```python
from build123d import *

# Parameters (mm, degrees)
SKETCH1_W           = 106
SKETCH1_H           = 106
BOSS_EXTRUDE1_DEPTH = 10
CUT_EXTRUDE9_DEPTH  = 1.5
SKETCH18_W          = 106
SKETCH18_H          = 106
SKETCH18_W_2        = 100
SKETCH18_H_2        = 100
CUT_EXTRUDE14_DEPTH = 10
SKETCH20_R          = 1
CUT_EXTRUDE15_DEPTH = 8
CUT_EXTRUDE16_START = -8
SKETCH21_R          = 1
CUT_EXTRUDE16_DEPTH = 8
SKETCH23_W          = 100
SKETCH23_H          = 100
SKETCH23_W_2        = 98
SKETCH23_H_2        = 98
CUT_EXTRUDE17_DEPTH = 10
SKETCH17_W          = 26.25282414
SKETCH17_H          = 10
CUT_EXTRUDE19_DEPTH = 10
FILLET2_R           = 3
FILLET3_R           = 3
FILLET4_R           = 2
SKETCH26_R          = 1.5
CUT_EXTRUDE20_DEPTH = 10
SKETCH27_R          = 2.5
CUT_EXTRUDE21_DEPTH = 2


with BuildPart() as part:
    # Sketch1 → Boss-Extrude1 (new body)
    with BuildSketch(Plane(origin=(0, 0, 0), x_dir=(1, 0, 0), z_dir=(0, 1, 0))):
        Rectangle(SKETCH1_W, SKETCH1_H)
    extrude(amount=BOSS_EXTRUDE1_DEPTH)

    # Sketch12 → Cut-Extrude9 (cut)
    with BuildSketch(Plane(origin=(53, 0, 0), x_dir=(0, 0, -1), z_dir=(1, 0, 0))):
        with BuildLine():
            ThreePointArc((-17.75, 5), (-18.262563133, 6.237436867), (-19.5, 6.75))
            Line((-19.5, 6.75), (-19.5, 3.25))
            ThreePointArc((-19.5, 3.25), (-18.262563133, 3.762563133), (-17.75, 5))
        make_face()
        with BuildLine():
            Line((-19.5, 3.25), (-19.5, 6.75))
            ThreePointArc((-19.5, 6.75), (-21.25, 5), (-19.5, 3.25))
        make_face()
        with BuildLine():
            ThreePointArc((21.25, 5), (20.737436867, 6.237436867), (19.5, 6.75))
            Line((19.5, 6.75), (19.5, 3.25))
            ThreePointArc((19.5, 3.25), (20.737436867, 3.762563133), (21.25, 5))
        make_face()
        with BuildLine():
            Line((19.5, 3.25), (19.5, 6.75))
            ThreePointArc((19.5, 6.75), (17.75, 5), (19.5, 3.25))
        make_face()
    extrude(amount=-CUT_EXTRUDE9_DEPTH, mode=Mode.SUBTRACT)

    # Sketch18 → Cut-Extrude14 (cut)
    with BuildSketch(Plane.XZ):
        Rectangle(SKETCH18_W, SKETCH18_H)
        Rectangle(SKETCH18_W_2, SKETCH18_H_2, mode=Mode.SUBTRACT)
    extrude(amount=-CUT_EXTRUDE14_DEPTH, mode=Mode.SUBTRACT)

    # Sketch20 → Cut-Extrude15 (cut)
    with BuildSketch(Plane(origin=(50, 0, 0), x_dir=(0, 0, -1), z_dir=(1, 0, 0))):
        with Locations((19.5, 5)):
            Circle(SKETCH20_R)
        with Locations((-19.5, 5)):
            Circle(SKETCH20_R)
    extrude(amount=-CUT_EXTRUDE15_DEPTH, mode=Mode.SUBTRACT)

    # Sketch21 → Cut-Extrude16 (cut)
    with BuildSketch(Plane.ZY.offset(50).offset(CUT_EXTRUDE16_START)):
        with Locations(Location((19.5, 5, 0), (0, 0, 180))):
            Circle(SKETCH21_R)
        with Locations(Location((-19.5, 5, 0), (0, 0, 180))):
            Circle(SKETCH21_R)
    extrude(amount=CUT_EXTRUDE16_DEPTH, mode=Mode.SUBTRACT)

    # Sketch23 → Cut-Extrude17 (cut)
    with BuildSketch(Plane.XZ):
        Rectangle(SKETCH23_W, SKETCH23_H)
        Rectangle(SKETCH23_W_2, SKETCH23_H_2, mode=Mode.SUBTRACT)
    extrude(amount=-CUT_EXTRUDE17_DEPTH, mode=Mode.SUBTRACT)

    # Sketch17 → Cut-Extrude19 (cut)
    with BuildSketch(Plane.XZ):
        Polygon((-40.464466094, 44), (0, 3.535533906), (40.464466094, 44), (17.869219367, 44), (17.869219367, 29), (-17.869219367, 29), (-17.869219367, 44), align=None)
        with Locations((0, 39)):
            Rectangle(SKETCH17_W, SKETCH17_H)
        Polygon((44, -40.464466094), (44, 40.464466094), (3.535533906, 0), align=None)
        Polygon((-3.535533906, 0), (-44, 40.464466094), (-44, -40.464466094), align=None)
        Polygon((17.869219367, -44), (40.464466094, -44), (0, -3.535533906), (-40.464466094, -44), (-17.869219367, -44), (-17.869219367, -29), (17.869219367, -29), align=None)
        with Locations((0, -39)):
            Rectangle(SKETCH17_W, SKETCH17_H)
    extrude(amount=-CUT_EXTRUDE19_DEPTH, mode=Mode.SUBTRACT)

    # Fillet2
    fillet2_edges = [part.edges().sort_by_distance(p)[0] for p in [
        (40.464466094, 5, 44),
        (0, 5, 3.535533906),
        (-40.464466094, 5, 44),
        (44, 5, 40.464466094),
        (3.535533906, 5, 0),
        (44, 5, -40.464466094),
        (-44, 5, -40.464466094),
        (-44, 5, 40.464466094),
        (-3.535533906, 5, 0),
        (-40.464466094, 5, -44),
        (0, 5, -3.535533906),
        (40.464466094, 5, -44),
    ]]
    fillet(fillet2_edges, radius=FILLET2_R)

    # Fillet3
    fillet3_edges = [part.edges().sort_by_distance(p)[0] for p in [
        (17.869219367, 5, 29),
        (17.869219367, 5, 44),
        (-17.869219367, 5, 44),
        (-17.869219367, 5, 29),
        (17.869219367, 5, -44),
        (17.869219367, 5, -29),
        (-17.869219367, 5, -29),
        (-17.869219367, 5, -44),
    ]]
    fillet(fillet3_edges, radius=FILLET3_R)

    # Fillet4
    fillet4_edges = [part.edges().sort_by_distance(p)[0] for p in [
        (13.12641207, 5, 34),
        (-13.12641207, 5, 34),
        (-13.12641207, 5, 44),
        (13.12641207, 5, 44),
        (13.12641207, 5, -44),
        (-13.12641207, 5, -44),
        (-13.12641207, 5, -34),
        (13.12641207, 5, -34),
    ]]
    fillet(fillet4_edges, radius=FILLET4_R)

    # Sketch26 → Cut-Extrude20 (cut)
    with BuildSketch(Plane(origin=(0, 10, 0), x_dir=(1, 0, 0), z_dir=(0, 1, 0))):
        with Locations(Location((44, -44, 0), (0, 0, 270))):
            Circle(SKETCH26_R)
        with Locations(Location((-44, -44, 0), (0, 0, 270))):
            Circle(SKETCH26_R)
        with Locations(Location((44, 44, 0), (0, 0, 270))):
            Circle(SKETCH26_R)
        with Locations(Location((-44, 44, 0), (0, 0, 270))):
            Circle(SKETCH26_R)
    extrude(amount=-CUT_EXTRUDE20_DEPTH, mode=Mode.SUBTRACT)

    # Sketch27 → Cut-Extrude21 (cut)
    with BuildSketch(Plane(origin=(0, 10, 0), x_dir=(1, 0, 0), z_dir=(0, 1, 0))):
        with Locations(Location((44, -44, 0), (0, 0, 270))):
            Circle(SKETCH27_R)
        with Locations(Location((-44, -44, 0), (0, 0, 270))):
            Circle(SKETCH27_R)
        with Locations(Location((-44, 44, 0), (0, 0, 270))):
            Circle(SKETCH27_R)
        with Locations(Location((44, 44, 0), (0, 0, 270))):
            Circle(SKETCH27_R)
    extrude(amount=-CUT_EXTRUDE21_DEPTH, mode=Mode.SUBTRACT)


solid = part.part
```
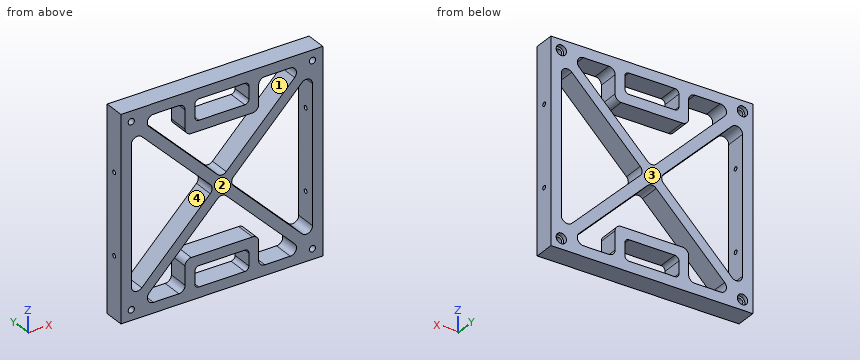
The model under review builds one solid part; all positions refer to its coordinate system, in mm. Face numbers are marked on the shaded views. A direction names the side the tool comes from. Round coordinates to 2 decimals unless told otherwise and drop trailing zeros. Order: outer loops, then holes, each group sorted by start corner. A loop starts at its lowest first (then second) coordinate and runs counter-clockwise, first axis right, second up. Notation, with made-up numbers: (34, 34.5) -> (92, 34.5) arc R8 cw to (92, 45.5) -> close; hole circle Ø11 at (80, 2). An arc over 180 degrees is marked (long way). One line per item, written item: value. Start each with the question number.
Q1. Mouldability with a two-part tool opening along X and no side actions: class the marked faces 3 and 4 as released by +X, released by -X, zero draft, split by the parting line, or undercut.
Q2. Take a section at D-D (y = 1.75). Count the separate pieces of the cut face and the enclosed holes in it, and give its area (3 significant figures).
Q3. Take a section at A-A (x = 0). Write out the cut boundary in (y, z).
Q4. Clearance check with flat-ended pins moving along their axes: pin 1 Ø2.5 at (y, z) = (5, -19.5) entering from -X; pin 2 Ø4 at (x, z) = (-44, 44) entering from +Y. State where each tip first meets the part, or that it passes through.
Q5. Wall thickness on line 1 (Z direction, x = -26.5, y = 1); line 2 (X direction, y = 3.75, z = -38.5); line 3 (Z direction, x = 33.5, y = 4.25): over which ranges is each line inside the solid? List them lowest first.
Q6. Take a section at C-C (x = -24). Write out the cut boundary in (y, z), and give its area (3 significant figures).
Q7. Take a section at B-B (z = -8). Write out the cut boundary in (x, y).
Q8. Machinability: for the marked faces 1 and 2, which of the approach directions +Z, -Z, +X, -X, +Y, -Y give a long, thin tool a straight path to every point of the face, cutting with its end or side? Answer none if there is none.
Reported:
1. face 3: zero draft
1. face 4: undercut
2. separate pieces: 1
2. enclosed holes: 10
2. area: 3,680 mm2
3. outline: (0, -49) -> (10, -49) -> (10, -44) -> (0, -44) -> close; (0, -34) -> (10, -34) -> (10, -29) -> (0, -29) -> close; (0, -4.78) -> (10, -4.78) -> (10, 4.78) -> (0, 4.78) -> close; (0, 29) -> (10, 29) -> (10, 34) -> (0, 34) -> close; (0, 44) -> (10, 44) -> (10, 49) -> (0, 49) -> close
4. pin 1: stops at x = -49
4. pin 2: stops at y = 8
5. line 1: z = -49 to -44, -30.04 to -22.96, 22.96 to 30.04, 44 to 49
5. line 2: x = -49 to -34.96, -17.87 to -13.13, 13.13 to 17.87, 34.96 to 49
5. line 3: z = -49 to -43.99, -37.04 to -29.96, 29.96 to 37.04, 43.99 to 49
6. outline: (0, -49) -> (10, -49) -> (10, -44) -> (0, -44) -> close; (0, -27.54) -> (10, -27.54) -> (10, -20.46) -> (0, -20.46) -> close; (0, 20.46) -> (10, 20.46) -> (10, 27.54) -> (0, 27.54) -> close; (0, 44) -> (10, 44) -> (10, 49) -> (0, 49) -> close
6. area: 241 mm2
7. outline: (-49, 0) -> (-44, 0) -> (-44, 10) -> (-49, 10) -> close; (-11.54, 0) -> (-4.46, 0) -> (-4.46, 10) -> (-11.54, 10) -> close; (4.46, 0) -> (11.54, 0) -> (11.54, 10) -> (4.46, 10) -> close; (44, 0) -> (49, 0) -> (49, 10) -> (44, 10) -> close
8. face 1: +Y, -Y
8. face 2: +Z, -Z, +X, -X, -Y
